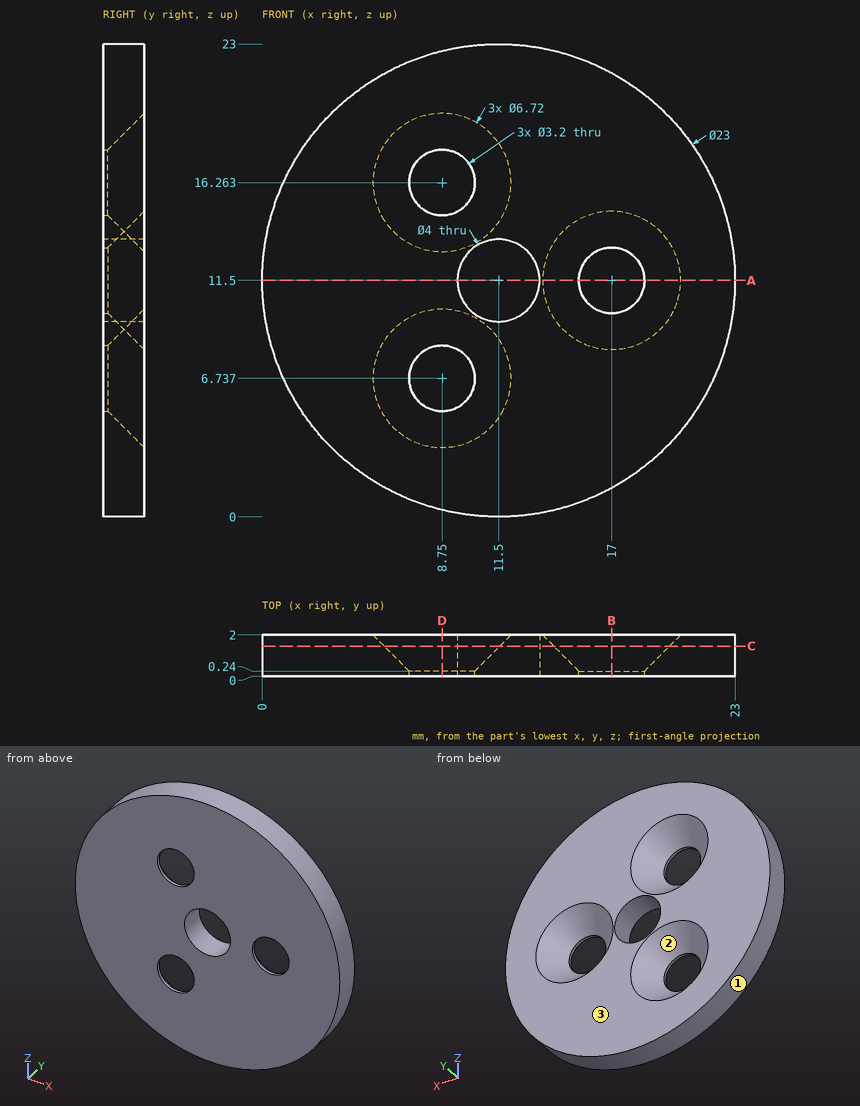
Geometry check sheet. Reference: drawing and pictorial views, mm from the part's lowest x, y, z. Give positions to 0.01 mm unless a question says otherwise; leave off trailing zeros. Order: outer loops, then holes, each group sorted by start corner. A loop starts at its lowest first (then second) coordinate and runs counter-clockwise, first axis right, second up. Notation, with made-up numbers: M 13,85 L 37,85 A13 cw 37,106 Z; hole C 64,61 d5. An arc over 180 degrees is marked long. Use one line per item in the form item = value. Start each with the question number.
Q1. Section check B-B (x = 17). Enter the section's corners in (y, z), then the cut area to 3 significant figures.
Q2. Section check A-A (z = 11.5). Enter the section's corners in (x, y), then the cut area to 3 significant figures.
Q3. Mould release check, pull along X, two halves, no side actions. Record for the marked faces 1, 2 and 3: +X half, -X half, draft (parallel to the pull), parting line (faces both ways), or undercut.
Q4. Go/stop test with a flat-tipped pin: pin 1 Ø3.5 at (x, z) = (8.75, 16.26) entering from +Y. Record where the tip stops, or that it passes through.
Q5. Scan lines: line 1 along X through (y, z) = (0.1, 11.5); line 2 along Z through (x, y) = (11.5, 1.05); line 3 along Z through (x, y) = (7.5, 0.1) (1 decimal). Record each from-to range of solid material in increasing order. Write a range as [from, to].
Q6. Section check D-D (x = 8.75). Enter the section's corners in (y, z), then the cut area to 3 significant figures.
Q7. Section check C-C (y = 1.45). Enter the section's corners in (x, z).
Evaluation:
q1.outline = M 0,1.4 L 2,1.4 L 2,8.14 L 0.24,9.9 L 0,9.9 Z; M 0,13.1 L 0.24,13.1 L 2,14.86 L 2,21.6 L 0,21.6 Z
q1.area = 30.9 mm2
q2.outline = M 0,0 L 9.5,0 L 9.5,2 L 0,2 Z; M 13.5,0 L 15.4,0 L 15.4,0.24 L 13.64,2 L 13.5,2 Z; M 18.6,0 L 23,0 L 23,2 L 20.36,2 L 18.6,0.24 Z
q2.area = 28.5 mm2
q3.face_1 = parting line
q3.face_2 = undercut
q3.face_3 = draft
q4.pin_1 = 0.39
q5.line_1 = [0, 9.5], [13.5, 15.4], [18.6, 23]
q5.line_2 = [0, 9.5], [13.5, 23]
q5.line_3 = [0.7, 5.7], [7.7, 15.3], [17.3, 22.3]
q6.outline = M 0,0.33 L 2,0.33 L 2,3.38 L 0.24,5.14 L 0,5.14 Z; M 0,8.34 L 0.24,8.34 L 2,10.1 L 2,12.9 L 0.24,14.66 L 0,14.66 Z; M 0,17.86 L 0.24,17.86 L 2,19.62 L 2,22.67 L 0,22.67 Z
q6.area = 25.7 mm2
q7.outline = C 11.5,11.5 d23; hole C 8.75,6.74 d5.62; hole C 8.75,16.26 d5.62; hole C 11.5,11.5 d4; hole C 17,11.5 d5.62
